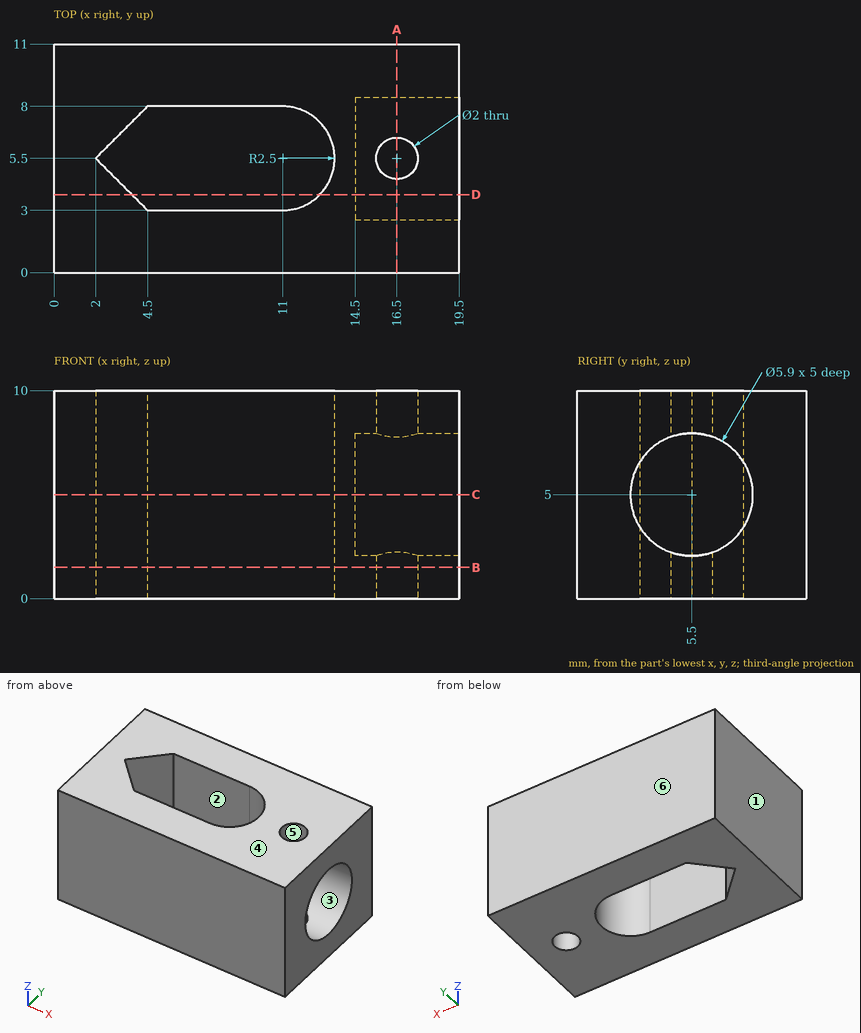
Input: dimensioned drawing with shaded views. Units: mm. Origin: part minimum x, y, z. A direction names the side the tool comes from. Give positions to 0.01 mm unless a question says otherwise; leave off trailing zeros. Write each loop counter-clockwise with the first axis right and the second up, starting at its lowest first coordinate (ties: lowest second). Pieces come first, ordered by that corner, then holes. Notation, with made-up numbers: M 37,27.25 L 76,27.25 A25 cw 76,49.25 Z; hole C 22.25,-35 d3. An arc over 180 degrees is marked long. Return JSON: item names as keys, results as strings. Group by question number.
1) Cut plane B-B, the plane z = 1.5. Output: boundary loops of the cut face in (x, y).
2) Pin query (flat end, axial travel): P1, Ø1.5, axis at y = 6, z = 7, coming from the +X side; P2, Ø1.6, axis at x = 16.5, y = 5.5, coming from the +Z side. Return the tip coordinate at first contact, or that it passes through.
3) Material intervals for line 1 along Y through (x, z) = (17.7, 5); line 2 along Y through (x, z) = (6.75, 8.75); line 3 along Z through (x, y) = (16.25, 4.25), sorted ascending. Write a range as [from, to].
4) Pull-direction query (Y, two-part tool) for the marked faces 4, 5 and 6; classes: pulls with the +Y half, pulls with the -Y half, needs draft (parallel to the pull), parting line crosses it, or undercut.
5) Cut plane D-D, the plane y = 3.75. Output: boundary loops of the cut face in (x, z).
6) Cut plane A-A, the plane x = 16.5. Output: boundary loops of the cut face in (y, z), plus the area to 3 significant figures.
7) Set-up query: the marked faces 1, 2 and 3. Return all of +Z, -Z, +X, -X, +Y, -Y with unobstructed straight access to the full face (end or side cutting, diameter ignored); none if empty.
8) Cut plane C-C, the plane z = 5. Output: boundary loops of the cut face in (x, y), plus the area to 3 significant figures.
Recorded:
{
 "1": {"outline": "M 0,0 L 19.5,0 L 19.5,11 L 0,11 Z; hole M 2,5.5 L 4.5,3 L 11,3 A2.5 ccw 11,8 L 4.5,8 Z; hole C 16.5,5.5 d2"},
 "2": {"P1": "stops at x = 14.5", "P2": "passes through"},
 "3": {"line 1": "y = [0, 2.55], [8.45, 11]", "line 2": "y = [0, 3], [8, 11]", "line 3": "z = [0, 2.33], [7.67, 10]"},
 "4": {"face 4": "needs draft", "face 5": "undercut", "face 6": "pulls with the +Y half"},
 "5": {"outline": "M 0,0 L 3.75,0 L 3.75,10 L 0,10 Z; M 12.79,0 L 19.5,0 L 19.5,2.63 L 14.5,2.63 L 14.5,7.37 L 19.5,7.37 L 19.5,10 L 12.79,10 Z"},
 "6": {"outline": "M 0,0 L 4.5,0 L 4.5,2.22 A2.95 cw 4.5,7.78 L 4.5,10 L 0,10 Z; M 6.5,0 L 11,0 L 11,10 L 6.5,10 L 6.5,7.78 A2.95 cw 6.5,2.22 Z", "area": "74.2 mm²"},
 "7": {"face 1": "+Z, -Z, -X, +Y, -Y", "face 2": "+Z, -Z", "face 3": "+X"},
 "8": {"outline": "M 0,0 L 19.5,0 L 19.5,2.55 L 14.5,2.55 L 14.5,8.45 L 19.5,8.45 L 19.5,11 L 0,11 Z; hole M 2,5.5 L 4.5,3 L 11,3 A2.5 ccw 11,8 L 4.5,8 Z", "area": "136 mm²"}
}
